Read the model definition and answer for the solid it produces. Units are mm, in the model's axes. Face numbers are marked on the shaded views. A direction names the side the tool comes from. Give positions to 0.01 mm unless a question says otherwise; leave off trailing zeros. Order: outer loops, then holes, each group sorted by start corner. A loop starts at its lowest first (then second) coordinate and runs counter-clockwise, first axis right, second up. Notation, with made-up numbers: (63, -22) -> (113, -22) arc R4 ccw to (113, -17) -> close; hole circle Ø2 at (89.25, 83.25). An arc over 180 degrees is marked (long way). Use one line per item in the form item = value.
```python
from build123d import *

# Parameters (mm, degrees)
F1_DEPTH     = 25.4
F2_W         = 15.1525349356
F2_H         = 13.7750366703
F3_DEPTH     = 18.288
F4_W         = 6.4649451524
F4_H         = 13.3289596997
F5_DEPTH     = 22.4028
F7_T1_DEPTH  = 25.1356456429
F7_T3_DEPTH  = 13.3289596997
F7_T8_DEPTH  = 50.5356473019
F7_T14_DEPTH = 50.5356473019
F8_W         = 0.189450098
F8_H         = 7.1646480085
F6_W         = 6.2150303274
F6_H         = 25.1356456429
F9_DEPTH     = 5.6896
F11_DEPTH    = 65.1764


# Not quite as in the source:
# - a fillet or chamfer that OpenCascade refuses, or shapes differently, is made with other operations: its cross-section is extruded or revolved along the edge and cut away or added


with BuildPart() as f1:
    # F0 (on Front) → F1 (new body)
    with BuildSketch(Plane.XZ):
        Polygon((0, 25.1356456429), (0, 0), (25.3690239042, 0), (25.3781564534, 25.1356456429), align=None)
    extrude(amount=F1_DEPTH)

    # F2 (on face) → F3 (cut)
    with BuildSketch(Plane.XY.offset(25.1356456429)):
        with Locations((12.512326939, -11.9383647107)):
            Rectangle(F2_W, F2_H)
    extrude(amount=-F3_DEPTH, mode=Mode.SUBTRACT)

    # F4 (on face) → F5 (join)
    with BuildSketch(Plane.XY.offset(25.1356456429)):
        with Locations((12.3413000256, -11.9561098982)):
            Rectangle(F4_W, F4_H)
    extrude(amount=-F5_DEPTH)

    # F7: fillet of radius 5.08 on 6 edges, made by hand

    # F7_s2 → F7_t1 (cut)
    with BuildSketch(Plane.XY):
        with BuildLine():
            ThreePointArc((0, -20.32), (1.4878975516, -23.9121024484), (5.08, -25.4))
            Line((5.08, -25.4), (5.08, -25.5016))
            Line((5.08, -25.5016), (-0.1016, -25.5016))
            Line((-0.1016, -25.5016), (-0.1016, -20.32))
            Line((-0.1016, -20.32), (0, -20.32))
        make_face()
        with BuildLine():
            ThreePointArc((0, -5.08), (1.4878975516, -1.4878975516), (5.08, 0))
            Line((5.08, 0), (5.08, 0.1016))
            Line((5.08, 0.1016), (-0.1016, 0.1016))
            Line((-0.1016, 0.1016), (-0.1016, -5.08))
            Line((-0.1016, -5.08), (0, -5.08))
        make_face()
    extrude(amount=F7_T1_DEPTH, mode=Mode.SUBTRACT)

    # F7_s4 → F7_t3 (cut)
    with BuildSketch(Plane.XZ.offset(5.2916300483)):
        with BuildLine():
            ThreePointArc((9.1088274494, 20.0556456429), (10.596725001, 23.6477480913), (14.1888274494, 25.1356456429))
            Line((14.1888274494, 25.1356456429), (14.1888274494, 25.2372456429))
            Line((14.1888274494, 25.2372456429), (9.0072274494, 25.2372456429))
            Line((9.0072274494, 25.2372456429), (9.0072274494, 20.0556456429))
            Line((9.0072274494, 20.0556456429), (9.1088274494, 20.0556456429))
        make_face()
        with BuildLine():
            ThreePointArc((15.5737726018, 20.0556456429), (14.0858750502, 23.6477480913), (10.4937726018, 25.1356456429))
            Line((10.4937726018, 25.1356456429), (10.4937726018, 25.2372456429))
            Line((10.4937726018, 25.2372456429), (15.6753726018, 25.2372456429))
            Line((15.6753726018, 25.2372456429), (15.6753726018, 20.0556456429))
            Line((15.6753726018, 20.0556456429), (15.5737726018, 20.0556456429))
        make_face()
    extrude(amount=F7_T3_DEPTH, mode=Mode.SUBTRACT)


with BuildPart() as f7_tool6:
    # F7_s7 → F7_t8 (new body)
    with BuildSketch(Plane(origin=(-0.0046109493, 0, -12.6907818203), x_dir=(0, 1, 0), z_dir=(0.0003633306, 0, 0.999999934))):
        with BuildLine():
            ThreePointArc((-25.4, -20.2890222297), (-23.9121024484, -23.8811246782), (-20.32, -25.3690222297))
            Line((-20.32, -25.3690222297), (-20.32, -25.4706222297))
            Line((-20.32, -25.4706222297), (-25.5016, -25.4706222297))
            Line((-25.5016, -25.4706222297), (-25.5016, -20.2890222297))
            Line((-25.5016, -20.2890222297), (-25.4, -20.2890222297))
        make_face()
    extrude(amount=F7_T8_DEPTH)

    split(bisect_by=Plane.XY.offset(25.1356456429), keep=Keep.BOTTOM)

    split(bisect_by=Plane.XY, keep=Keep.TOP)


with BuildPart() as f1_1:
    add(f1.part)

    # F7_t5: cut F7_tool6
    add(f7_tool6.part, mode=Mode.SUBTRACT)


with BuildPart() as f7_tool12:
    # F7_s13 → F7_t14 (new body)
    with BuildSketch(Plane(origin=(-0.0046109493, 0, -12.6907818203), x_dir=(0, 1, 0), z_dir=(0.0003633306, 0, 0.999999934))):
        with BuildLine():
            ThreePointArc((0, -20.2890222297), (-1.4878975516, -23.8811246782), (-5.08, -25.3690222297))
            Line((-5.08, -25.3690222297), (-5.08, -25.4706222297))
            Line((-5.08, -25.4706222297), (0.1016, -25.4706222297))
            Line((0.1016, -25.4706222297), (0.1016, -20.2890222297))
            Line((0.1016, -20.2890222297), (0, -20.2890222297))
        make_face()
    extrude(amount=F7_T14_DEPTH)

    split(bisect_by=Plane.XY.offset(25.1356456429), keep=Keep.BOTTOM)

    split(bisect_by=Plane.XY, keep=Keep.TOP)


with BuildPart() as f1_2:
    add(f1_1.part)

    # F7_t11: cut F7_tool12
    add(f7_tool12.part, mode=Mode.SUBTRACT)

    # F8 (on face) + F6 (on face) → F9 (cut)
    with BuildSketch(Plane.XZ.offset(25.4)):
        with Locations((15.687267526, 12.4311717227)):
            Rectangle(F8_W, F8_H)
    with BuildSketch(Plane.XZ.offset(25.4)):
        with Locations((12.4850273132, 12.5678228214)):
            Rectangle(F6_W, F6_H)
    extrude(amount=-F9_DEPTH, mode=Mode.SUBTRACT)

    # F10 (on face) → F11 (cut)
    with BuildSketch(Plane.XZ):
        Polygon((15.2985183522, 3.9248324286), (15.2985183522, 15.5202150633), (15.2985183522, 19.5378263631), (9.7349686548, 19.5378263631), (9.7349686548, 3.9248324286), align=None)
    extrude(amount=F11_DEPTH, mode=Mode.SUBTRACT)


solid = f1_2.part
```
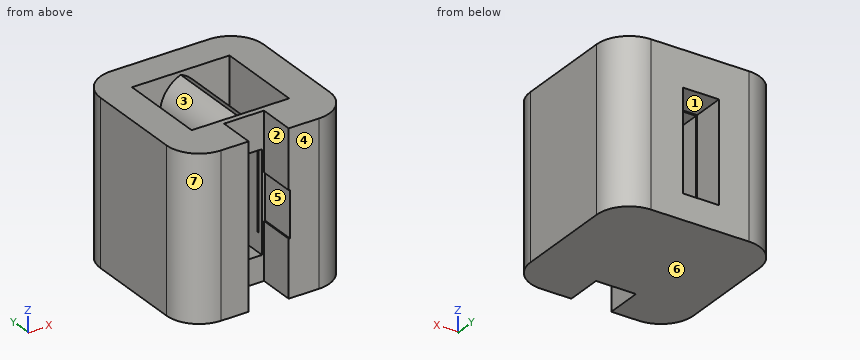
Item 1: Determine the mould class of the marked faces 5, 6 and 7 for opening direction X: +X half, -X half, draft (parallel to the pull), parting line (faces both ways), or undercut.
Checks:
face_5 = undercut
face_6 = draft
face_7 = -X half
Item 2: Straight lines are drawn through the part: L1, parallel to X at y = -18.5, z = 11; L2, parallel to Y at x = 20, z = 18; L3, parallel to Y at x = 15, z = 21. For each, find the intervals that lie inside material, in ascending order. Write a range as from..to.
Checks:
L1 = 0..4.94, 9.11..9.73, 15.3..15.57, 20.09..25.37
L2 = -25.4..-18.83, -5.05..0
L3 = -19.71..-18.83, -18.62..-5.29, -5.05..0
Item 3: The part is cut by section B-B on y = -22. Give the vertices of the cut face in (x, z), and give its area (3 significant figures).
Checks:
outline = (0.29, 0) -> (9.38, 0) -> (9.38, 25.14) -> (0.29, 25.14) -> close; (15.59, 0) -> (25.08, 0) -> (25.09, 25.14) -> (15.59, 25.14) -> (15.59, 16.01) -> (15.78, 16.01) -> (15.78, 8.85) -> (15.59, 8.85) -> close
area = 466 mm²
Item 4: Which of the six approach directions +Z, -Z, +X, -X, +Y, -Y give full straight-line access (tool end or side, diameter ignored) to the marked faces 1, 2, 3 and 4?
Checks:
face_1 = +Y, -Y
face_2 = +Z, -Z, -Y
face_3 = +Z
face_4 = +Z, -Z, +X, -X, -Y
Item 5: Given pin 1 Ø2.5 at (x, y) = (18.5, -9) entering from +Z; pin 2 Ø1.7 at (y, z) = (-23, 20) entering from -X; pin 3 Ø4.5 at (y, z) = (-7.5, 15.5) entering from +X, each flat-ended and moving along its own axis, determine where each tip first touches the part or whether it passes through.
Checks:
pin_1 = 6.85
pin_2 = 0.34
pin_3 = 25.38
Item 6: The part is cut by section D-D on x = 13.75. Give the vertices of the cut face in (y, z).
Checks:
outline = (-19.71, 0) -> (0, 0) -> (0, 3.92) -> (-19.71, 3.92) -> close; (-19.71, 19.54) -> (-18.83, 19.54) -> (-18.83, 25.14) -> (-19.71, 25.14) -> close; (-18.62, 19.54) -> (-5.29, 19.54) -> (-5.29, 23.95) -> (-18.62, 23.95) -> close; (-5.05, 19.54) -> (0, 19.54) -> (0, 25.14) -> (-5.05, 25.14) -> close
Item 7: The part is cut by section A-A on y = -6.25. Give the vertices of the cut face in (x, z).
Checks:
outline = (0, 0) -> (25.37, 0) -> (25.38, 25.14) -> (20.09, 25.14) -> (20.09, 6.85) -> (15.57, 6.85) -> (15.57, 20.06) arc R5.08 ccw to (12.34, 24.79) arc R5.08 ccw to (9.11, 20.06) -> (9.11, 6.85) -> (4.94, 6.85) -> (4.94, 25.14) -> (0, 25.14) -> close; hole (9.73, 3.92) -> (15.3, 3.92) -> (15.3, 19.54) -> (9.73, 19.54) -> close
Item 8: The part is cut by section C-C on x = 19. Give the vertices of the cut face in (y, z), and give its area (3 significant figures).
Checks:
outline = (-25.4, 0) -> (0, 0) -> (0, 25.14) -> (-5.05, 25.14) -> (-5.05, 6.85) -> (-18.83, 6.85) -> (-18.83, 25.14) -> (-25.4, 25.14) -> close
area = 387 mm²
